```python
from build123d import *

# Parameters (mm, degrees)
F0_R     = 20.955
F1_DEPTH = 25.4
F3_DEPTH = 25.4


with BuildPart() as f1:
    # F0 (on Right) → F1 (new body)
    with BuildSketch(Plane.YZ):
        Circle(F0_R)
    extrude(amount=F1_DEPTH)

    # F2 (on face) → F3 (cut)
    with BuildSketch(Plane.YZ.offset(25.4)):
        Polygon((0, -18.923), (5.499261, -18.923), (10.998523, -9.398), (5.499261, 0.127), (-5.499261, 0.127), (-10.998523, -9.398), (-5.499261, -18.923), align=None)
    extrude(amount=-F3_DEPTH, mode=Mode.SUBTRACT)


solid = f1.part
```
For this review, take the finished solid that the model builds, in its own axes (mm). A direction names the side the tool comes from. Round coordinates to 2 decimals unless told otherwise and drop trailing zeros. Write each loop counter-clockwise with the first axis right and the second up, starting at its lowest first coordinate (ties: lowest second). Pieces come first, ordered by that corner, then holes. Notation, with made-up numbers: (31, 37.5) -> (43, 37.5) arc R30 ccw to (43, 68.5) -> close; hole circle Ø8 at (67, 45). An arc over 180 degrees is marked (long way). One line per question, with ' | ' between items. Start each with the question number.
(1) Add section D-D, the plane z = 14.5. Write out the cut boundary in (x, y), plus the area to 3 significant figures.
(2) Add section B-B, the plane y = 0. Write out the cut boundary in (x, z) (3 decimals), plus the area to 3 significant figures.
(3) Add section C-C, the plane z = -3.5. Write out the cut boundary in (x, y).
(4) Add section A-A, the plane x = 5.75. Write out the cut boundary in (y, z) (3 decimals).
(5) For line 1 along Y through (x, z) = (19.75, -15); line 2 along Z through (x, y) = (23, -2.5); line 3 along Y through (x, z) = (16, -6), list the stretches that pass through material, from the lowest coordinate up. Write a range as from..to.
(6) Insertion check: P1, Ø1, axis at x = 12, y = 9.5, coming from the -Z side; P2, Ø4, axis at x = 9, z = -8, coming from the -Y side; P3, Ø6, axis at x = 22.5, z = -6.5, coming from the +Y side; P4, Ø3, axis at x = 6, z = 0.5, coming from the -Y side (3 decimals). Each pin has a flat end and moves straight along its axis. Give the tip position at first contact, or say it passes through.
(7) Tool access review of faces 1 (the face through (25.4, 0, 5)), 2 (the face through (12.878, 8.287, -4.702)): name each direction out of +Z, -Z, +X, -X, +Y, -Y from which nothing blocks a thin tool from reaching the whole face with its end or side.
Answer list:
1) outline: (0, -15.13) -> (25.4, -15.13) -> (25.4, 15.13) -> (0, 15.13) -> close | area: 769 mm²
2) outline: (0, -20.955) -> (25.4, -20.955) -> (25.4, -18.923) -> (0, -18.923) -> close; (0, 0.127) -> (25.4, 0.127) -> (25.4, 20.955) -> (0, 20.955) -> close | area: 581 mm²
3) outline: (0, -20.66) -> (25.4, -20.66) -> (25.4, -7.59) -> (0, -7.59) -> close; (0, 7.59) -> (25.4, 7.59) -> (25.4, 20.66) -> (0, 20.66) -> close
4) outline: circle Ø41.91 at (0, 0); hole (-10.999, -9.398) -> (-5.499, -18.923) -> (5.499, -18.923) -> (10.999, -9.398) -> (5.499, 0.127) -> (-5.499, 0.127) -> close
5) line 1: -14.63..-7.76, 7.76..14.63 | line 2: -20.81..-18.92, 0.13..20.81 | line 3: -20.08..-9.04, 9.04..20.08
6) P1: z = -18.92 | P2: y = -20.08 | P3: y = 20.66 | P4: y = -20.955
7) face 1: +Z, -Z, +X, +Y, -Y | face 2: +X, -X
